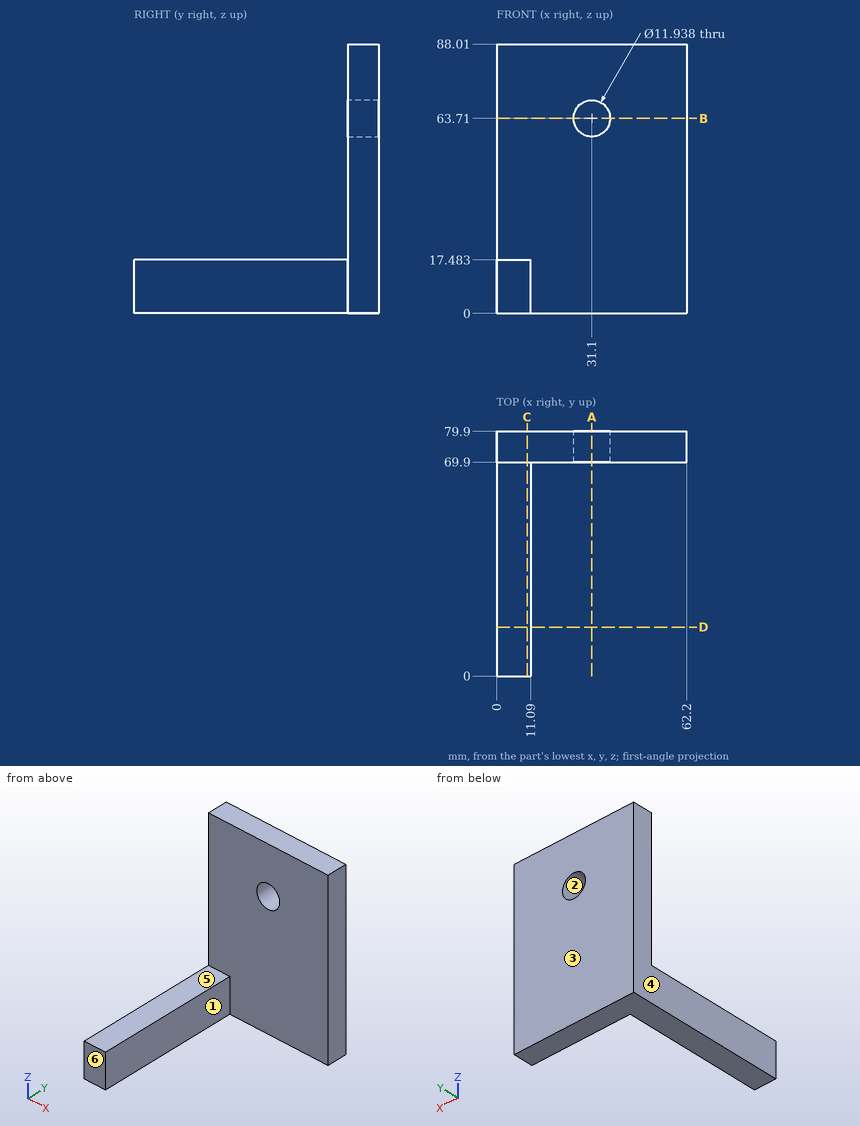
Here's the drawing with two shaded views (mm, measured from the low corner). I have some questions. A direction names the side the tool comes from. Coordinates: 2 decimals unless noted, no trailing zeros. Loops run counter-clockwise (first coordinate to the right, second up) from the corner with the lowest first, then second, coordinate; pieces in that order, holes last.
Item 1: I'm going to push flat-ended pins straight in: pin 1 (4 mm diameter, centred on x = 44.5, z = 61, fed in from -Y); pin 2 (8 mm diameter, centred on y = 52.5, z = 12.5, fed in from +X); pin 3 (3 mm diameter, centred on x = 42.5, y = 69, fed in from -Z); pin 4 (12 mm diameter, centred on x = 4.5, y = 49.5, fed in from +Z). Where does each tip first touch, or does it pass through?
Answers below:
pin 1: stops at y = 69.9
pin 2: stops at x = 11.09
pin 3: stops at z = 0
pin 4: stops at z = 17.48
Item 2: Please list where these lines run through material, in increasing order: L1, parallel to X at y = 72, z = 63.71; L2, parallel to X at y = 35, z = 4; L3, parallel to Y at x = 48, z = 6.5.
Answers below:
L1: x = 0 to 25.13, 37.07 to 62.2
L2: x = 0 to 11.09
L3: y = 69.9 to 79.9
Item 3: Which directions (+Z, -Z, +X, -X, +Y, -Y) give clear straight access to the entire face, cutting with the end or side of a thin tool? Please do the marked faces 5 and 6.
Answers below:
face 5: +Z, +X, -X, -Y
face 6: +Z, -Z, +X, -X, -Y
Item 4: Suppose I cut it at A-A (x = 31.1). Please give me the cut outline in (y, z), then the cut area to 3 significant figures.
Answers below:
outline: (69.9, 0) - (79.9, 0) - (79.9, 57.74) - (69.9, 57.74) - close; (69.9, 69.68) - (79.9, 69.68) - (79.9, 88.01) - (69.9, 88.01) - close
area: 761 mm2
Item 5: Suppose I cut it at D-D (y = 16). Please give me the cut outline in (x, z).
Answers below:
outline: (0, 0) - (11.09, 0) - (11.09, 17.48) - (0, 17.48) - close
Item 6: Suppose I cut it at C-C (x = 10). Please give me the cut outline in (y, z).
Answers below:
outline: (0, 0) - (79.9, 0) - (79.9, 88.01) - (69.9, 88.01) - (69.9, 17.48) - (0, 17.48) - close
Item 7: If we mould it in two halves opening along X, with no side actions, what happens to the marked faces 1, 2, 3 and 4? For each: released by +X, released by -X, zero draft, split by the parting line, or undercut.
Answers below:
face 1: released by +X
face 2: undercut
face 3: zero draft
face 4: released by -X
Item 8: Suppose I cut it at B-B (z = 63.71). Please give me the cut outline in (x, y), then the cut area to 3 significant figures.
Answers below:
outline: (0, 69.9) - (25.13, 69.9) - (25.13, 79.9) - (0, 79.9) - close; (37.07, 69.9) - (62.2, 69.9) - (62.2, 79.9) - (37.07, 79.9) - close
area: 503 mm2
